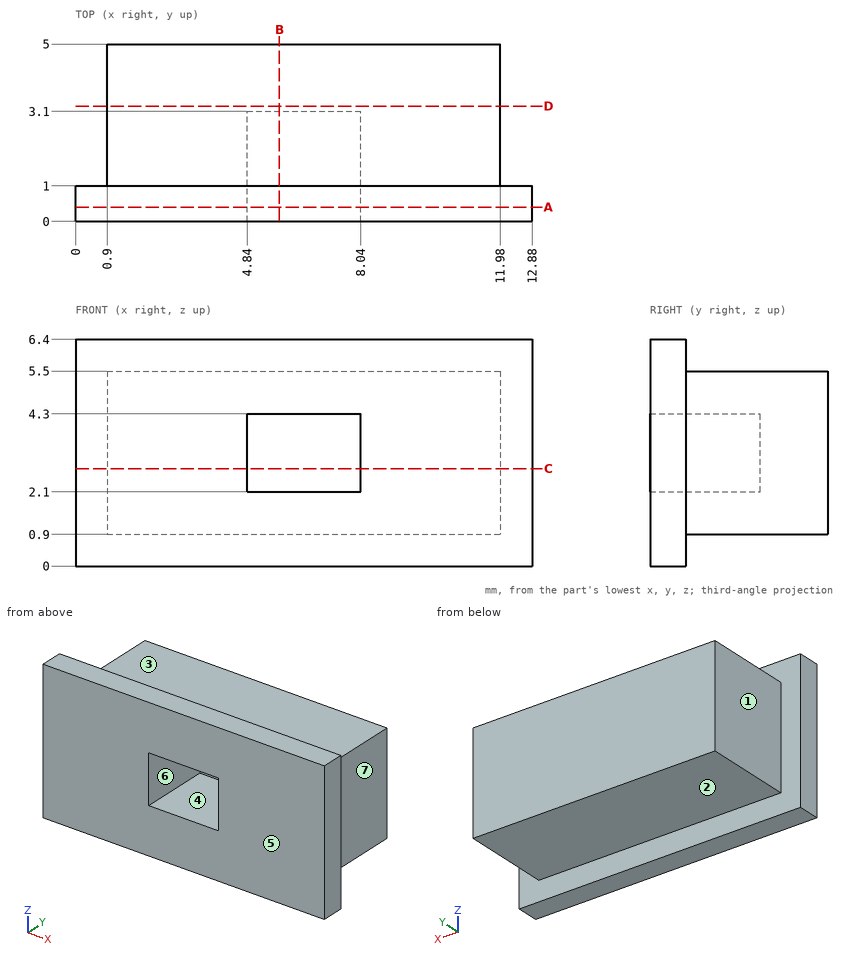
Drawing for the job (mm, zero at the part's lowest x, y, z). A direction names the side the tool comes from. Round coordinates to 2 decimals unless told otherwise and drop trailing zeros. Order: outer loops, then holes, each group sorted by start corner. A loop starts at its lowest first (then second) coordinate and runs counter-clockwise, first axis right, second up.
Item 1: Saw through at C-C on z = 2.75. Write the cut outline in (x, y), then the cut area to 3 significant figures.
Item 2: Tool access for the marked faces 1, 2 and 3: list every direction of +Z, -Z, +X, -X, +Y, -Y with a clear straight run to the whole face (end or side of a thin tool).
Item 3: Probe line 1 along X through (y, z) = (1.2, 3.25); line 2 along Z through (x, y) = (5.5, 1.6); line 3 along Z through (x, y) = (5.75, 4.2). List the from-to ranges inside material, lowest first.
Item 4: Saw through at B-B on x = 5.75. Write the cut outline in (y, z).
Item 5: Mould opens along X. For the marked faces 4, 5, 6 and 7 say: pulls with the +X half, pulls with the -X half, needs draft (parallel to the pull), parting line crosses it, or undercut.
Item 6: Saw through at D-D on y = 3.25. Write the cut outline in (x, z).
Item 7: Saw through at A-A on y = 0.4. Write the cut outline in (x, z), then the cut area to 3 significant figures.
Item 8: Pin check, flat tips, straight feed: pin 1 (2 mm diameter, centred on x = 8, y = 3, fed in from +Z); pin 2 (0.7 mm diameter, centred on x = 5.5, z = 3.5, fed in from -Y); pin 3 (2 mm diameter, centred on y = 3.5, z = 3, fed in from +X). Stop position of each tip, or through.
Reported:
1. outline: (0, 0) - (4.84, 0) - (4.84, 3.1) - (8.04, 3.1) - (8.04, 0) - (12.88, 0) - (12.88, 1) - (11.98, 1) - (11.98, 5) - (0.9, 5) - (0.9, 1) - (0, 1) - close
1. area: 47.3 mm2
2. face 1: +Z, -Z, -X, +Y
2. face 2: -Z, +X, -X, +Y
2. face 3: +Z, +X, -X, +Y
3. line 1: x = 0.9 to 4.84, 8.04 to 11.98
3. line 2: z = 0.9 to 2.1, 4.3 to 5.5
3. line 3: z = 0.9 to 5.5
4. outline: (0, 0) - (1, 0) - (1, 0.9) - (5, 0.9) - (5, 5.5) - (1, 5.5) - (1, 6.4) - (0, 6.4) - (0, 4.3) - (3.1, 4.3) - (3.1, 2.1) - (0, 2.1) - close
5. face 4: undercut
5. face 5: needs draft
5. face 6: undercut
5. face 7: pulls with the +X half
6. outline: (0.9, 0.9) - (11.98, 0.9) - (11.98, 5.5) - (0.9, 5.5) - close
7. outline: (0, 0) - (12.88, 0) - (12.88, 6.4) - (0, 6.4) - close; hole (4.84, 2.1) - (8.04, 2.1) - (8.04, 4.3) - (4.84, 4.3) - close
7. area: 75.4 mm2
8. pin 1: stops at z = 5.5
8. pin 2: stops at y = 3.1
8. pin 3: stops at x = 11.98
